Geometry: final body of the model. Coordinates: model frame, mm. Give positions to 0.01 mm unless a question says otherwise; leave off trailing zeros. Write each loop counter-clockwise with the first axis right and the second up, starting at its lowest first coordinate (ties: lowest second). Pieces come first, ordered by that corner, then holes.
Q1. Section B-B (x = 0). Return the cut outline in (y, z).
Q2. Section A-A (z = 10). Return the cut outline in (x, y).
Q3. Line query: line 1 (Z direction, x = -10, y = 0); line 2 (Y direction, x = 0, z = 9); line 3 (Y direction, x = 11, z = 10.5). Output: solid intervals per line, ascending.
Q4. Pin query (flat end, axial travel): pin 1 Ø4 at (y, z) = (7, 7.5) entering from -X; pin 2 Ø1.5 at (y, z) = (-9, 2.5) entering from -X; pin 3 Ø3 at (y, z) = (0, 6) entering from -X; pin 4 Ø3 at (x, y) = (-16, -15.5) entering from +Z. Return the tip coordinate at first contact, or that it passes through.
Q5. Section C-C (y = 0). Return the cut outline in (x, z).
Q6. Mould query, pull axis Y, two halves, no side actions, for faces 1 (the cylindrical face through (19.33, 5.14, 5.92)), 2 (the cylindrical face through (19.31, -5.21, 5.92)), 3 (the cylindrical face through (-19.37, -1.68, 4.58)), 4 (the flat face through (0, 5, 12)). Classes: +Y half, -Y half, draft (parallel to the pull), parting line (faces both ways), or undercut.
Q7. Section D-D (z = 6). Return the cut outline in (x, y).
from build123d import *

# Parameters (mm, degrees)
SKETCH_R           = 20
PAD_DEPTH          = 12
SKETCH001_R        = 4
POCKET_DEPTH       = 127.655658
POLARPATTERN_COUNT = 12
SKETCH002_R        = 4.1
POCKET001_DEPTH    = 12.001
SKETCH003_R        = 1.9
POCKET002_DEPTH    = 26


with BuildPart() as part:
    # Sketch → Pad (new body)
    with BuildSketch(Plane.XY):
        Circle(SKETCH_R)
    extrude(amount=PAD_DEPTH)

    # Sketch001 (on Face2 of Pad) → Pocket (cut, through all)
    with BuildSketch(Plane(origin=(0, 0, 0), x_dir=(1, 0, 0), z_dir=(0, 0, -1))):
        with Locations((0, 23)):
            Circle(SKETCH001_R)
    pocket = extrude(amount=-POCKET_DEPTH, mode=Mode.SUBTRACT)

    # PolarPattern: Pocket ×12 about axis
    polarpattern_axis = Axis((0, 0, 0), (0, 0, -1))
    for i in range(1, POLARPATTERN_COUNT):
        add(pocket.rotate(polarpattern_axis, i * 360 / POLARPATTERN_COUNT), mode=Mode.SUBTRACT)

    # Sketch002 (on Face2 of PolarPattern) → Pocket001 (cut, through all)
    with BuildSketch(Plane(origin=(0, 0, 0), x_dir=(1, 0, 0), z_dir=(0, 0, -1))):
        Circle(SKETCH002_R)
    extrude(amount=-POCKET001_DEPTH, mode=Mode.SUBTRACT)

    # Sketch003 → Pocket002 (cut)
    with BuildSketch(Plane.YZ):
        with Locations((0, 6)):
            Circle(SKETCH003_R)
    extrude(amount=-POCKET002_DEPTH, mode=Mode.SUBTRACT)


solid = part.part
Computed:
1. outline: (-19, 0) - (-4.1, 0) - (-4.1, 12) - (-19, 12) - close; (4.1, 0) - (19, 0) - (19, 12) - (4.1, 12) - close
2. outline: (-19.85, -2.46) arc R20 ccw to (-18.42, -7.79) arc R4 cw to (-15.96, -12.06) arc R20 ccw to (-12.06, -15.96) arc R4 cw to (-7.79, -18.42) arc R20 ccw to (-2.46, -19.85) arc R4 cw to (2.46, -19.85) arc R20 ccw to (7.79, -18.42) arc R4 cw to (12.06, -15.96) arc R20 ccw to (15.96, -12.06) arc R4 cw to (18.42, -7.79) arc R20 ccw to (19.85, -2.46) arc R4 cw to (19.85, 2.46) arc R20 ccw to (18.42, 7.79) arc R4 cw to (15.96, 12.06) arc R20 ccw to (12.06, 15.96) arc R4 cw to (7.79, 18.42) arc R20 ccw to (2.46, 19.85) arc R4 cw to (-2.46, 19.85) arc R20 ccw to (-7.79, 18.42) arc R4 cw to (-12.06, 15.96) arc R20 ccw to (-15.96, 12.06) arc R4 cw to (-18.42, 7.79) arc R20 ccw to (-19.85, 2.46) arc R4 cw to start; hole circle Ø8.2 at (0, 0)
3. line 1: z = 0 to 4.1, 7.9 to 12
3. line 2: y = -19 to -4.1, 4.1 to 19
3. line 3: y = -15.95 to 15.95
4. pin 1: stops at x = -19.36
4. pin 2: stops at x = -17.59
4. pin 3: stops at x = 3.82
4. pin 4: passes through
5. outline: (-19, 0) - (-4.1, 0) - (-4.1, 4.1) - (-19, 4.1) - close; (-19, 7.9) - (-4.1, 7.9) - (-4.1, 12) - (-19, 12) - close; (4.1, 0) - (19, 0) - (19, 12) - (4.1, 12) - close
6. face 1: +Y half
6. face 2: -Y half
6. face 3: undercut
6. face 4: draft
7. outline: (-19.85, -2.46) arc R20 ccw to (-18.42, -7.79) arc R4 cw to (-15.96, -12.06) arc R20 ccw to (-12.06, -15.96) arc R4 cw to (-7.79, -18.42) arc R20 ccw to (-2.46, -19.85) arc R4 cw to (2.46, -19.85) arc R20 ccw to (7.79, -18.42) arc R4 cw to (12.06, -15.96) arc R20 ccw to (15.96, -12.06) arc R4 cw to (18.42, -7.79) arc R20 ccw to (19.85, -2.46) arc R4 cw to (19.85, 2.46) arc R20 ccw to (18.42, 7.79) arc R4 cw to (15.96, 12.06) arc R20 ccw to (12.06, 15.96) arc R4 cw to (7.79, 18.42) arc R20 ccw to (2.46, 19.85) arc R4 cw to (-2.46, 19.85) arc R20 ccw to (-7.79, 18.42) arc R4 cw to (-12.06, 15.96) arc R20 ccw to (-15.96, 12.06) arc R4 cw to (-18.42, 7.79) arc R20 ccw to (-19.85, 2.46) arc R4 cw to (-19.48, 1.9) - (-3.63, 1.9) arc R4.1 cw (long way) to (-3.63, -1.9) - (-19.48, -1.9) arc R4 cw to start
